from build123d import *

# Parameters (mm, degrees)
SKETCH1_R           = 127
BOSS_EXTRUDE1_DEPTH = 6.35
SKETCH2_R           = 2.54
CUT_EXTRUDE1_DEPTH  = 7.35
CIRPATTERN1_COUNT   = 4


with BuildPart() as part:
    # Sketch1 → Boss-Extrude1 (new body)
    with BuildSketch(Plane.XY):
        Circle(SKETCH1_R)
    extrude(amount=BOSS_EXTRUDE1_DEPTH)

    # Sketch2 → Cut-Extrude1 (cut, through all)
    with BuildSketch(Plane.XY.offset(6.35)):
        Circle(SKETCH2_R)
    extrude(amount=-CUT_EXTRUDE1_DEPTH, mode=Mode.SUBTRACT)

    # Sketch5 → #10 Clearance Hole1 (revolve, cut)
    with BuildSketch(Plane(origin=(0, 12.7, 6.35), x_dir=(0, -1, 0), z_dir=(1, 0, 0))):
        Polygon((0, 0), (0, 11.058816902), (2.5527, 9.525), (2.5527, 0), align=None)
    f_10_clearance_hole1 = revolve(axis=Axis((0, 12.7, 12.7), (0, 0, -1)), mode=Mode.SUBTRACT)

    # CirPattern1: #10 Clearance Hole1 ×4 about axis
    cirpattern1_axis = Axis((0, 0, 0), (0, 0, 1))
    for i in range(1, CIRPATTERN1_COUNT):
        add(f_10_clearance_hole1.rotate(cirpattern1_axis, i * 360 / CIRPATTERN1_COUNT), mode=Mode.SUBTRACT)


solid = part.part
Geometry check sheet. Reference: the model listing, model coordinates, mm. Give positions to 0.01 mm unless a question says otherwise; leave off trailing zeros. Write each loop counter-clockwise with the first axis right and the second up, starting at its lowest first coordinate (ties: lowest second). Pieces come first, ordered by that corner, then holes.
1) Cross-section at A-A (z = 1.75). Record the boundary of the cut face in (x, y), plus the area to 3 significant figures.
Values follow:
outline: circle Ø254 at (0, 0); hole circle Ø5.11 at (-12.7, 0); hole circle Ø5.11 at (0, -12.7); hole circle Ø5.11 at (0, 12.7); hole circle Ø5.08 at (0, 0); hole circle Ø5.11 at (12.7, 0)
area: 50,600 mm2
2) Cross-section at C-C (y = -61). Record the boundary of the cut face in (x, z).
Values follow:
outline: (-111.39, 0) - (111.39, 0) - (111.39, 6.35) - (-111.39, 6.35) - close
3) Thickness scan on line 1 (Y direction, x = 0, z = 3.5); line 2 (X direction, y = 12.7, z = 4.75); line 3 (X direction, y = 1, z = 2.5). Record the ranges inside material, lowest first.
Values follow:
line 1: y = -127 to -15.25, -10.15 to -2.54, 2.54 to 10.15, 15.25 to 127
line 2: x = -126.36 to -2.55, 2.55 to 126.36
line 3: x = -127 to -15.05, -10.35 to -2.33, 2.33 to 10.35, 15.05 to 127
4) Cross-section at B-B (x = 75.5). Record the boundary of the cut face in (y, z), plus the area to 3 significant figures.
Values follow:
outline: (-102.12, 0) - (102.12, 0) - (102.12, 6.35) - (-102.12, 6.35) - close
area: 1,300 mm2
